```python
from build123d import *

# Parameters (mm, degrees)
SKETCH1_R           = 1.6
BOSS_EXTRUDE1_DEPTH = 1.5
CUT_EXTRUDE1_DEPTH  = 1.5
BOSS_EXTRUDE2_DEPTH = 1.5
FILLET1_R           = 4


with BuildPart() as part:
    # Sketch1 → Boss-Extrude1 (new body)
    with BuildSketch(Plane.XY):
        Polygon((5, 59), (-32, 72.466898668), (-32, 56), (-32, 0), (-32, -16.466898668), (5, -3), align=None)
        Circle(SKETCH1_R, mode=Mode.SUBTRACT)
        with Locations((-28, 0)):
            Circle(SKETCH1_R, mode=Mode.SUBTRACT)
        with Locations((0, 56)):
            Circle(SKETCH1_R, mode=Mode.SUBTRACT)
        with Locations((-28, 56)):
            Circle(SKETCH1_R, mode=Mode.SUBTRACT)
    extrude(amount=BOSS_EXTRUDE1_DEPTH)

    # Sketch2 → Cut-Extrude1 (cut)
    with BuildSketch(Plane.XY.offset(1.5)):
        Polygon((5, 59), (-43.875673323, 59), (-43.875673323, 79.145449881), (45.915909875, 71.47170947), align=None)
        Polygon((5, -3), (-36.907564214, -3), (-45.551547665, -23.435700668), (23.159300381, -21.407010674), align=None)
    extrude(amount=-CUT_EXTRUDE1_DEPTH, mode=Mode.SUBTRACT)

    # Sketch3 → Boss-Extrude2 (add)
    with BuildSketch(Plane.XY.offset(1.5)):
        Polygon((-32, 59), (5, 68.91412012), (5, 59), align=None)
        Polygon((5, -3), (5, -12.91412012), (-32, -3), align=None)
    extrude(amount=-BOSS_EXTRUDE2_DEPTH)

    # Fillet1
    fillet1_edges = [part.edges().sort_by_distance(p)[0] for p in [
        (-32, 59, 0.75),
        (-32, -3, 0.75),
        (5, 68.91412012, 0.75),
        (5, -12.91412012, 0.75),
    ]]
    fillet(fillet1_edges, radius=FILLET1_R)


solid = part.part
```
Build history of the part. All positions in model axes, mm. Round coordinates to 2 decimals unless told otherwise and drop trailing zeros. Write each loop counter-clockwise with the first axis right and the second up, starting at its lowest first coordinate (ties: lowest second). Pieces come first, ordered by that corner, then holes. Notation, with made-up numbers: (-28, -3) - (3, -3) arc R18 cw to (3, 14) - close; hole circle Ø2 at (-16.75, -21). An arc over 180 degrees is marked (long way). Write each question's results on one line, items separated by ' | '. Start each with the question number.
Item 1: Saw through at D-D (x = -17.5). Write the cut outline in (y, z), and give its area (3 significant figures).
Item 2: Wall check: L1, parallel to Y at x = -28, z = 0.55; L2, parallel to Y at x = -21, z = 0.5; L3, parallel to Y at x = -14.5, z = 1.25. Give the ranges that are in metal, low to high. Write a range as [from, to].
Item 3: Mould opens along Y. For faces 1 (the face through (-1.27, -0.97, 0.74)), 2 (the face through (3.4, 66.9, 0.7)), 3 (the face through (-31.151, -2.395, 0.76)), 4 (the face through (-29.6, 56.07, 0.74)) say: pulls with the +Y half, pulls with the -Y half, needs draft (parallel to the pull), parting line crosses it, or undercut.
Item 4: Saw through at B-B (x = -28). Write the cut outline in (y, z).
Item 5: Saw through at A-A (z = 1). Write the cut outline in (x, y).
Item 6: Saw through at C-C (x = -7). Write the cut outline in (y, z).
Results are:
1) outline: (-6.89, 0) - (62.89, 0) - (62.89, 1.5) - (-6.89, 1.5) - close | area: 105 mm²
2) L1: y = [-4.07, -1.6], [1.6, 54.4], [57.6, 60.07] | L2: y = [-5.95, 61.95] | L3: y = [-7.69, 63.69]
3) face 1: undercut | face 2: pulls with the +Y half | face 3: pulls with the -Y half | face 4: undercut
4) outline: (-4.07, 0) - (-1.6, 0) - (-1.6, 1.5) - (-4.07, 1.5) - close; (1.6, 0) - (54.4, 0) - (54.4, 1.5) - (1.6, 1.5) - close; (57.6, 0) - (60.07, 0) - (60.07, 1.5) - (57.6, 1.5) - close
5) outline: (-32, 0.07) arc R4 ccw to (-29.04, -3.79) - (-0.04, -11.56) arc R4 ccw to (5, -7.7) - (5, 63.7) arc R4 ccw to (-0.04, 67.56) - (-29.04, 59.79) arc R4 ccw to (-32, 55.93) - close; hole circle Ø3.2 at (-28, 0); hole circle Ø3.2 at (-28, 56); hole circle Ø3.2 at (0, 0); hole circle Ø3.2 at (0, 56)
6) outline: (-9.7, 0) - (65.7, 0) - (65.7, 1.5) - (-9.7, 1.5) - close
